The model under review builds one solid part; all positions refer to its coordinate system, in mm. A direction names the side the tool comes from. Give positions to 0.01 mm unless a question says otherwise; leave off trailing zeros. Write each loop counter-clockwise with the first axis right and the second up, starting at its lowest first coordinate (ties: lowest second). Pieces come first, ordered by that corner, then holes. Notation, with made-up numbers: (-27, 43) - (-21, 43) arc R8 cw to (-21, 56) - close; hole circle Ø4 at (56.25, -24.5). An arc over 180 degrees is marked (long way). Write item = value, one per line.
```python
from build123d import *

# Parameters (mm, degrees)
F1_DEPTH  = 12.7
F3_DEPTH  = 101.6
F5_DEPTH  = 38.101
F6_W      = 42.559474
F6_H      = 49.497269
F7_DEPTH  = 38.101
F8_R      = 2
F9_DEPTH  = 5
F10_R     = 5
F10_R_2   = 2
F11_DEPTH = 0.5
F12_R     = 1.8
F13_DEPTH = 5
F14_R     = 1
F16_DEPTH = 12.7
F17_R     = 5.08
F18_SIZE  = 5.08


with BuildPart() as f1:
    # F0 (on Right) → F1 (new body)
    with BuildSketch(Plane.YZ):
        Polygon((0, 101.6), (0, 0), (52.753847, 0), (101.6, 0), (150.446153, 0), (203.2, 0), (203.2, 101.6), (101.6, 101.6), align=None)
    extrude(amount=F1_DEPTH)

    # F2 (on face) → F3 (join, through all)
    with BuildSketch(Plane(origin=(0, 0, 0), x_dir=(1, 0, 0), z_dir=(0, 0, -1))):
        with BuildLine():
            Line((12.7, 0), (12.7, -203.2))
            ThreePointArc((12.7, -203.2), (38.1, -101.6), (12.7, 0))
        make_face()
    extrude(amount=-F3_DEPTH)

    # F4 (on face) → F5 (cut, through all)
    with BuildSketch(Plane(origin=(0, 0, 0), x_dir=(0, -1, 0), z_dir=(-1, 0, 0))):
        with BuildLine():
            Line((-101.6, 0), (-19.05, 0))
            ThreePointArc((-19.05, 0), (-59.240217, 14.225728), (-101.6, 19.05))
            Line((-101.6, 19.05), (-101.6, 0))
        make_face()
        with BuildLine():
            Line((-101.6, 0), (-101.6, 19.05))
            ThreePointArc((-101.6, 19.05), (-143.959783, 14.225728), (-184.15, 0))
            Line((-184.15, 0), (-101.6, 0))
        make_face()
    extrude(amount=-F5_DEPTH, mode=Mode.SUBTRACT)

    # F6 (on face) → F7 (cut, through all)
    with BuildSketch(Plane(origin=(0, 0, 0), x_dir=(0, -1, 0), z_dir=(-1, 0, 0))):
        with Locations((-221.472621, 114.174965)):
            Rectangle(F6_W, F6_H)
    extrude(amount=-F7_DEPTH, mode=Mode.SUBTRACT)

    # F8 (on face) → F9 (cut)
    with BuildSketch(Plane(origin=(0, 0, 0), x_dir=(1, 0, 0), z_dir=(0, 0, -1))):
        with Locations((11.1125, -6.35)):
            Circle(F8_R)
    extrude(amount=-F9_DEPTH, mode=Mode.SUBTRACT)

    # F10 (on face) → F11 (join)
    with BuildSketch(Plane(origin=(0, 0, 0), x_dir=(1, 0, 0), z_dir=(0, 0, -1))):
        with Locations((11.1125, -6.35)):
            Circle(F10_R)
        with Locations((11.1125, -6.35)):
            Circle(F10_R_2, mode=Mode.SUBTRACT)
    extrude(amount=F11_DEPTH)

    # F12 (on face) → F13 (join)
    with BuildSketch(Plane.XY.offset(101.6)):
        with Locations((11.1125, 6.35)):
            Circle(F12_R)
    extrude(amount=F13_DEPTH)

    # F14
    f14_edges = [f1.edges().sort_by_distance(p)[0] for p in [
        (9.3125, 6.35, 106.6),
    ]]
    fillet(f14_edges, radius=F14_R)

    # F15 (on face) → F16 (cut)
    with BuildSketch(Plane(origin=(0, 0, 0), x_dir=(0, -1, 0), z_dir=(-1, 0, 0))):
        Polygon((-100.096442, 101.6), (-188.996442, 101.6), (-188.996442, 0), (-100.096442, 0), (-11.196442, 0), (-11.196442, 101.6), align=None)
    extrude(amount=-F16_DEPTH, mode=Mode.SUBTRACT)

    # F17
    f17_edges = [f1.edges().sort_by_distance(p)[0] for p in [
        (0, 0, 50.8),
        (0, 11.196442, 50.8),
    ]]
    fillet(f17_edges, radius=F17_R)

    # F18
    f18_edges = [f1.edges().sort_by_distance(p)[0] for p in [
        (12.7, 101.6, 19.05),
    ]]
    chamfer(f18_edges, length=F18_SIZE)


solid = f1.part
```
1. For line 1 (Y direction, x = 9.5, z = 46); line 2 (Y direction, x = 7.5, z = 92.5); line 3 (Z direction, x = 14, y = 190), list the stretches that pass through material, from the lowest coordinate up. Write a range as from..to.
Findings below:
line_1 = 0..11.2, 189..203.2
line_2 = 0..11.2, 189..200.19
line_3 = 0..101.6
2. Take a section at B-B on z = 33.5. Give the boundary of the cut face in (x, y), and give its area (4 significant figures).
Findings below:
outline = (0, 5.08) arc R5.08 ccw to (5.08, 0) - (12.7, 0) arc R215.9 ccw to (12.7, 203.2) - (0, 203.2) - (0, 189) - (12.7, 189) - (12.7, 11.2) - (5.08, 11.2) arc R5.08 ccw to (0, 6.12) - close
area = 3,795 mm²
3. Take a section at A-A on x = 3. Give the boundary of the cut face in (y, z), and give its area (3 significant figures).
Findings below:
outline = (0.45, 0) - (10.75, 0) - (10.75, 101.6) - (0.45, 101.6) - close; (189, 0) - (203.2, 0) - (203.2, 89.43) - (200.19, 89.43) - (200.19, 101.6) - (189, 101.6) - close
area = 2,450 mm²
4. Take a section at C-C on x = 31.5. Give the boundary of the cut face in (y, z).
Findings below:
outline = (48.63, 11.45) arc R188.38 cw to (101.6, 19.05) arc R188.38 cw to (154.57, 11.45) - (154.57, 101.6) - (48.63, 101.6) - close
5. Insertion check: P1, Ø15, axis at x = 16, y = 194, coming from the -Z side; P2, Ø1.5, axis at x = 6.5, y = 202.5, coming from the +Z side; P3, Ø1.5, axis at y = 171.5, z = 91, coming from the -X side. Each pin has a flat end and moves straight along its axis. Give the tip position at first contact, or say it passes through.
Findings below:
P1 = 0
P2 = 89.43
P3 = 12.7
6. Draft analysis for pull direction Y (two halves, no side actions). For faces 1 (the flat face through (6, 203.2, 44)), 2 (the cylindrical face through (1.449, 1.528, 50.089)), 3 (the flat face through (13.3, 6.3, -0.5)), 4 (the flat face through (11, 6, 5)), state which applies: +Y half, -Y half, draft (parallel to the pull), parting line (faces both ways), or undercut.
Findings below:
face_1 = +Y half
face_2 = -Y half
face_3 = draft
face_4 = undercut
7. Machinability: for faces 5 (the flat face through (7, 200.193, 95)), 6 (the cylindrical face through (9.314, 6.429, 103.572)), 7 (the cylindrical face through (13.02, 5.75, 2.29)), 8 (the cylindrical face through (1.53, 9.75, 51.51)), 9 (the flat face through (8, 194, 0)), which of the approach directions +Z, -Z, +X, -X, +Y, -Y give a long, thin tool a straight path to every point of the face, cutting with its end or side? Answer none if there is none.
Findings below:
face_5 = +Z, +X, -X, +Y
face_6 = +Z
face_7 = -Z
face_8 = +Z, -Z, -X
face_9 = -Z, +X, -X, +Y
